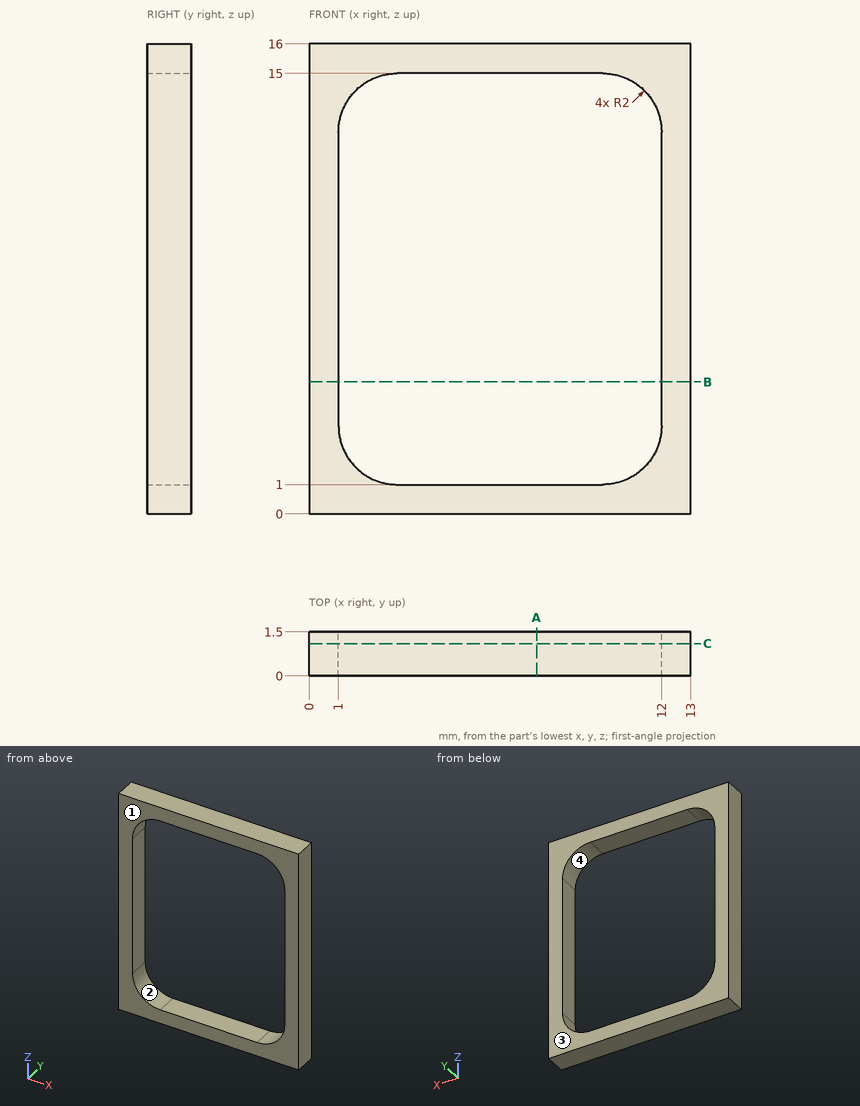
Job drawing, mm, ordinate dimensions from the low corner. One solid piece. A direction names the side the tool comes from. Coordinates: 2 decimals unless noted, no trailing zeros. Write each loop counter-clockwise with the first axis right and the second up, starting at its lowest first coordinate (ties: lowest second). Pieces come first, ordered by that corner, then holes.
Item 1: Mould opens along Z. For the marked faces 1 and 2 say: released by +Z, released by -Z, zero draft, split by the parting line, or undercut.
Item 2: Slice it at B-B (z = 4.5). Write the cut outline in (x, y).
Item 3: Slice it at A-A (x = 7.75). Write the cut outline in (y, z), and give its area (3 significant figures).
Item 4: Probe line 1 (X direction, y = 0.5, z = 8.25); line 2 (Z direction, x = 5.5, y = 1.25); line 3 (Z direction, x = 11, y = 0.9). List the from-to ranges inside material, lowest first.
Item 5: Pin check, flat tips, straight feed: pin 1 (4 mm diameter, centred on x = 10.5, z = 12.5, fed in from -Y); pin 2 (5 mm diameter, centred on x = 5.5, z = 9, fed in from -Y). Stop position of each tip, or through.
Item 6: Slice it at C-C (y = 1.1). Write the cut outline in (x, z), and give its area (3 significant figures).
Item 7: Which spindle directions (+Z, -Z, +X, -X, +Y, -Y) get a long thin tool onto all of the face, cutting with end or side? Do the marked faces 3 and 4. Say none if no direction does.
Results found:
1. face 1: zero draft
1. face 2: undercut
2. outline: (0, 0) - (1, 0) - (1, 1.5) - (0, 1.5) - close; (12, 0) - (13, 0) - (13, 1.5) - (12, 1.5) - close
3. outline: (0, 0) - (1.5, 0) - (1.5, 1) - (0, 1) - close; (0, 15) - (1.5, 15) - (1.5, 16) - (0, 16) - close
3. area: 3.00 mm2
4. line 1: x = 0 to 1, 12 to 13
4. line 2: z = 0 to 1, 15 to 16
4. line 3: z = 0 to 1.27, 14.73 to 16
5. pin 1: stops at y = 0
5. pin 2: passes through
6. outline: (0, 0) - (13, 0) - (13, 16) - (0, 16) - close; hole (1, 3) arc R2 ccw to (3, 1) - (10, 1) arc R2 ccw to (12, 3) - (12, 13) arc R2 ccw to (10, 15) - (3, 15) arc R2 ccw to (1, 13) - close
6. area: 57.4 mm2
7. face 3: +Z, -Z, +X, -X, +Y
7. face 4: +Y, -Y
